Work out the finished part from the listing and answer in its coordinate system (mm). Coordinates: 2 decimals unless noted, no trailing zeros. Loops run counter-clockwise (first coordinate to the right, second up) from the corner with the lowest first, then second, coordinate; pieces in that order, holes last. Notation, with made-up numbers: (78.5, -10) - (125.5, -10) arc R16 ccw to (125.5, 10) - close; hole circle Ø7 at (45, 84.5). An arc over 180 degrees is marked (long way). Write each question's results on one line, items separated by ' | '. Start each with the question number.
1. A cutting plane is placed at C-C on z = 3. Determine the outline of the cut face in (x, y).
2. Determine the mould class of faces 1 (the flat face through (38.1, -13, 0)), 2 (the cylindrical face through (1.58, -12.52, 10.77)), 3 (the flat face through (19, -13, 19.05)), 4 (the cylindrical face through (1.666, -12.522, -8.455)) for opening direction Z: released by +Z, released by -Z, zero draft, split by the parting line, or undercut.
3. This flat-tipped pin is pushed along its axis until it touches: P1, Ø3, axis at y = -19.5, z = -1.5, coming from the -X side. Where does it stop, or does it pass through?
4. A cutting plane is placed at B-B on z = -5.5. Determine the outline of the cut face in (x, y), then the cut area to 3 significant figures.
5. Find the intervals of material crossed by line 1 along X through (y, z) = (-22.5, -1); line 2 along Z through (x, y) = (2, -22.5), in increasing order. Write a range as [from, to].
from build123d import *

# Parameters (mm, degrees)
F0_W     = 38.1
F0_H     = 38.1
F1_DEPTH = 25.4
F3_DEPTH = 25.401


with BuildPart() as f1:
    # F0 (on Front) → F1 (new body)
    with BuildSketch(Plane.XZ):
        with Locations((19.05, 0)):
            Rectangle(F0_W, F0_H)
    extrude(amount=F1_DEPTH)

    # F2 (on Front) → F3 (cut, through all)
    with BuildSketch(Plane.XZ):
        with BuildLine():
            Line((2.222374, 9.23115), (2.222291, 9.177008))
            ThreePointArc((2.222291, 9.177008), (2.222497, 9.204079), (2.222374, 9.23115))
        make_face()
        with BuildLine():
            Line((2.197918, -6.655362), (2.222291, 9.177008))
            Line((2.222291, 9.177008), (2.222374, 9.23115))
            ThreePointArc((2.222374, 9.23115), (1.563161, 10.787384), (0, 11.43))
            Line((0, 11.43), (0, -9.2075))
            ThreePointArc((0, -9.2075), (1.684061, -8.435325), (2.197918, -6.655362))
        make_face()
    extrude(amount=F3_DEPTH, mode=Mode.SUBTRACT)


solid = f1.part
Values:
1) outline: (2.21, -25.4) - (38.1, -25.4) - (38.1, 0) - (2.21, 0) - close
2) face 1: zero draft | face 2: undercut | face 3: released by +Z | face 4: undercut
3) P1: x = 2.2
4) outline: (2.2, -25.4) - (38.1, -25.4) - (38.1, 0) - (2.2, 0) - close | area: 912 mm^2
5) line 1: [2.21, 38.1] | line 2: [-19.05, -7.95], [10.18, 19.05]
